from build123d import *
from OCP.BRepFilletAPI import BRepFilletAPI_MakeChamfer

# Parameters (mm, degrees)
SKETCH1_R                      = 20.575
SKETCH1_R_2                    = 18.575
BOSS_EXTRUDE1_DEPTH            = 20
BOSS_EXTRUDE2_START            = -1.95
SKETCH2_R                      = 35.575
SKETCH2_R_2                    = 20.575
BOSS_EXTRUDE2_DEPTH            = 1.95
CHAMFER2_SIZE                  = 2
CHAMFER2_SIZE2                 = 0.727940469
SKETCH3_W                      = 2
SKETCH3_H                      = 18
CUT_EXTRUDE1_DEPTH             = 0.8
CHAMFER3_SIZE                  = 2.197981936
CHAMFER3_SIZE_2                = 0.8
CIRPATTERN2_COUNT              = 6
CHAMFER3_OF_CIRPATTERN2_SIZE   = 2.197981936
CHAMFER3_OF_CIRPATTERN2_SIZE_2 = 0.8


with BuildPart() as part:
    # Sketch1 → Boss-Extrude1 (new body)
    with BuildSketch(Plane.XY):
        Circle(SKETCH1_R)
        Circle(SKETCH1_R_2, mode=Mode.SUBTRACT)
    extrude(amount=BOSS_EXTRUDE1_DEPTH)

    # Sketch2 → Boss-Extrude2 (add)
    with BuildSketch(Plane.XY.offset(20).offset(BOSS_EXTRUDE2_START)):
        Circle(SKETCH2_R)
        Circle(SKETCH2_R_2, mode=Mode.SUBTRACT)
    extrude(amount=BOSS_EXTRUDE2_DEPTH)

    # Chamfer2
    chamfer2_edges = [part.edges().sort_by_distance(p)[0] for p in [
        (-18.575, 0, 0),
        (-18.575, 0, 20),
    ]]
    chamfer2_side = [part.faces().sort_by_distance(p)[0] for p in [
        (-18.575, 0, 10),
    ]]
    chamfer(chamfer2_edges, length=CHAMFER2_SIZE, length2=CHAMFER2_SIZE2, reference=chamfer2_side[0])

    # Sketch3 → Cut-Extrude1 (cut)
    with BuildSketch(Plane.XY.offset(20)):
        with Locations((0, 27.575)):
            Rectangle(SKETCH3_W, SKETCH3_H)
    cut_extrude1 = extrude(amount=-CUT_EXTRUDE1_DEPTH, mode=Mode.SUBTRACT)

    # Chamfer3
    chamfer3_edges_1 = [part.edges().sort_by_distance(p)[0] for p in [
        (1, 27.418981343, 20),
    ]]
    chamfer3_side_1 = [part.faces().sort_by_distance(p)[0] for p in [
        (1.016, 27.418981343, 20),
    ]]
    chamfer3_edges_2 = [part.edges().sort_by_distance(p)[0] for p in [
        (-1, 27.418981343, 20),
    ]]
    chamfer3_side_2 = [part.faces().sort_by_distance(p)[0] for p in [
        (-1.016, 27.418981343, 20),
    ]]
    chamfer3 = BRepFilletAPI_MakeChamfer(part.part.solid().wrapped)
    for e in chamfer3_edges_1:
        chamfer3.Add(CHAMFER3_SIZE - 0.0001, CHAMFER3_SIZE_2 - 0.0001, e.wrapped, chamfer3_side_1[0].wrapped)
    for e in chamfer3_edges_2:
        chamfer3.Add(CHAMFER3_SIZE - 0.0001, CHAMFER3_SIZE_2 - 0.0001, e.wrapped, chamfer3_side_2[0].wrapped)
    add(Compound.cast(chamfer3.Shape()), mode=Mode.REPLACE)  # a hair under: the kernel refuses the full size

    # CirPattern2: Cut-Extrude1 ×6 about axis
    cirpattern2_axis = Axis((0, 0, 0), (0, 0, 1))
    for i in range(1, CIRPATTERN2_COUNT):
        add(cut_extrude1.rotate(cirpattern2_axis, i * 360 / CIRPATTERN2_COUNT), mode=Mode.SUBTRACT)

    # Chamfer3 of CirPattern2
    chamfer3_of_cirpattern2_edges_1 = [part.edges().sort_by_distance(p)[0] for p in [
        (-23.245534389, 14.575516075, 20),
    ]]
    chamfer3_of_cirpattern2_side_1 = [part.faces().sort_by_distance(p)[0] for p in [
        (-23.237534389, 14.589372482, 20),
    ]]
    chamfer3_of_cirpattern2_edges_2 = [part.edges().sort_by_distance(p)[0] for p in [
        (-24.245534389, 12.843465267, 20),
    ]]
    chamfer3_of_cirpattern2_side_2 = [part.faces().sort_by_distance(p)[0] for p in [
        (-24.245534389, 12.843465267, 19.984),
    ]]
    chamfer3_of_cirpattern2_edges_3 = [part.edges().sort_by_distance(p)[0] for p in [
        (-24.245534389, -12.843465267, 20),
    ]]
    chamfer3_of_cirpattern2_side_3 = [part.faces().sort_by_distance(p)[0] for p in [
        (-24.253534389, -12.829608861, 20),
    ]]
    chamfer3_of_cirpattern2_edges_4 = [part.edges().sort_by_distance(p)[0] for p in [
        (-23.245534389, -14.575516075, 20),
    ]]
    chamfer3_of_cirpattern2_side_4 = [part.faces().sort_by_distance(p)[0] for p in [
        (-23.245534389, -14.575516075, 19.984),
    ]]
    chamfer3_of_cirpattern2_edges_5 = [part.edges().sort_by_distance(p)[0] for p in [
        (-1, -27.418981343, 20),
    ]]
    chamfer3_of_cirpattern2_side_5 = [part.faces().sort_by_distance(p)[0] for p in [
        (-1.016, -27.418981343, 20),
    ]]
    chamfer3_of_cirpattern2_edges_6 = [part.edges().sort_by_distance(p)[0] for p in [
        (1, -27.418981343, 20),
    ]]
    chamfer3_of_cirpattern2_side_6 = [part.faces().sort_by_distance(p)[0] for p in [
        (1, -27.418981343, 19.984),
    ]]
    chamfer3_of_cirpattern2_edges_7 = [part.edges().sort_by_distance(p)[0] for p in [
        (23.245534389, -14.575516075, 20),
    ]]
    chamfer3_of_cirpattern2_side_7 = [part.faces().sort_by_distance(p)[0] for p in [
        (23.237534389, -14.589372482, 20),
    ]]
    chamfer3_of_cirpattern2_edges_8 = [part.edges().sort_by_distance(p)[0] for p in [
        (24.245534389, -12.843465267, 20),
    ]]
    chamfer3_of_cirpattern2_side_8 = [part.faces().sort_by_distance(p)[0] for p in [
        (24.245534389, -12.843465267, 19.984),
    ]]
    chamfer3_of_cirpattern2_edges_9 = [part.edges().sort_by_distance(p)[0] for p in [
        (24.245534389, 12.843465267, 20),
    ]]
    chamfer3_of_cirpattern2_side_9 = [part.faces().sort_by_distance(p)[0] for p in [
        (24.253534389, 12.829608861, 20),
    ]]
    chamfer3_of_cirpattern2_edges_10 = [part.edges().sort_by_distance(p)[0] for p in [
        (23.245534389, 14.575516075, 20),
    ]]
    chamfer3_of_cirpattern2_side_10 = [part.faces().sort_by_distance(p)[0] for p in [
        (23.245534389, 14.575516075, 19.984),
    ]]
    chamfer3_of_cirpattern2 = BRepFilletAPI_MakeChamfer(part.part.solid().wrapped)
    for e in chamfer3_of_cirpattern2_edges_1:
        chamfer3_of_cirpattern2.Add(CHAMFER3_OF_CIRPATTERN2_SIZE - 0.0001, CHAMFER3_OF_CIRPATTERN2_SIZE_2 - 0.0001, e.wrapped, chamfer3_of_cirpattern2_side_1[0].wrapped)
    for e in chamfer3_of_cirpattern2_edges_2:
        chamfer3_of_cirpattern2.Add(CHAMFER3_OF_CIRPATTERN2_SIZE_2 - 0.0001, CHAMFER3_OF_CIRPATTERN2_SIZE - 0.0001, e.wrapped, chamfer3_of_cirpattern2_side_2[0].wrapped)
    for e in chamfer3_of_cirpattern2_edges_3:
        chamfer3_of_cirpattern2.Add(CHAMFER3_OF_CIRPATTERN2_SIZE - 0.0001, CHAMFER3_OF_CIRPATTERN2_SIZE_2 - 0.0001, e.wrapped, chamfer3_of_cirpattern2_side_3[0].wrapped)
    for e in chamfer3_of_cirpattern2_edges_4:
        chamfer3_of_cirpattern2.Add(CHAMFER3_OF_CIRPATTERN2_SIZE_2 - 0.0001, CHAMFER3_OF_CIRPATTERN2_SIZE - 0.0001, e.wrapped, chamfer3_of_cirpattern2_side_4[0].wrapped)
    for e in chamfer3_of_cirpattern2_edges_5:
        chamfer3_of_cirpattern2.Add(CHAMFER3_OF_CIRPATTERN2_SIZE - 0.0001, CHAMFER3_OF_CIRPATTERN2_SIZE_2 - 0.0001, e.wrapped, chamfer3_of_cirpattern2_side_5[0].wrapped)
    for e in chamfer3_of_cirpattern2_edges_6:
        chamfer3_of_cirpattern2.Add(CHAMFER3_OF_CIRPATTERN2_SIZE_2 - 0.0001, CHAMFER3_OF_CIRPATTERN2_SIZE - 0.0001, e.wrapped, chamfer3_of_cirpattern2_side_6[0].wrapped)
    for e in chamfer3_of_cirpattern2_edges_7:
        chamfer3_of_cirpattern2.Add(CHAMFER3_OF_CIRPATTERN2_SIZE - 0.0001, CHAMFER3_OF_CIRPATTERN2_SIZE_2 - 0.0001, e.wrapped, chamfer3_of_cirpattern2_side_7[0].wrapped)
    for e in chamfer3_of_cirpattern2_edges_8:
        chamfer3_of_cirpattern2.Add(CHAMFER3_OF_CIRPATTERN2_SIZE_2 - 0.0001, CHAMFER3_OF_CIRPATTERN2_SIZE - 0.0001, e.wrapped, chamfer3_of_cirpattern2_side_8[0].wrapped)
    for e in chamfer3_of_cirpattern2_edges_9:
        chamfer3_of_cirpattern2.Add(CHAMFER3_OF_CIRPATTERN2_SIZE - 0.0001, CHAMFER3_OF_CIRPATTERN2_SIZE_2 - 0.0001, e.wrapped, chamfer3_of_cirpattern2_side_9[0].wrapped)
    for e in chamfer3_of_cirpattern2_edges_10:
        chamfer3_of_cirpattern2.Add(CHAMFER3_OF_CIRPATTERN2_SIZE_2 - 0.0001, CHAMFER3_OF_CIRPATTERN2_SIZE - 0.0001, e.wrapped, chamfer3_of_cirpattern2_side_10[0].wrapped)
    add(Compound.cast(chamfer3_of_cirpattern2.Shape()), mode=Mode.REPLACE)  # a hair under: the kernel refuses the full size


solid = part.part
Model file for the job. Use its own axes, mm. A direction names the side the tool comes from. Give positions to 0.01 mm unless a question says otherwise; leave off trailing zeros. Write each loop counter-clockwise with the first axis right and the second up, starting at its lowest first coordinate (ties: lowest second). Pieces come first, ordered by that corner, then holes. Notation, with made-up numbers: (-10.75, 2) -> (23.25, 2) arc R24 ccw to (23.25, 35) -> close; hole circle Ø11 at (64.25, -9). An arc over 180 degrees is marked (long way). Write item = value, one per line.
(1) Probe line 1 along Y through (x, z) = (0, 11) (3 decimals); line 2 along Z through (x, y) = (28.5, -15.5); line 3 along Z through (x, y) = (9, 29.5). List the from-to ranges inside material, lowest first.
Determined:
line_1 = -20.575 to -18.575, 18.575 to 20.575
line_2 = 18.05 to 19.2
line_3 = 18.05 to 20
(2) Mould opens along X. For faces 1 (the face through (-2.1, 27.2, 19.6)), 2 (the face through (11.06, 17.35, 8.9)), 3 (the face through (22.462, 15.41, 19.606)) say: released by +X, released by -X, zero draft, split by the parting line, or undercut.
Determined:
face_1 = undercut
face_2 = split by the parting line
face_3 = undercut
(3) Slice it at C-C, the plane z = 12.75. Give the cut face in (x, y) (3 decimals), then the cut area to 3 significant figures.
Determined:
outline = circle Ø41.15 at (0, 0); hole circle Ø37.15 at (0, 0)
area = 246 mm2
(4) Slice it at A-A, the plane y = 0. Give the cut face in (x, z) (3 decimals), then the cut area to 3 significant figures.
Determined:
outline = (-35.575, 18.05) -> (-20.575, 18.05) -> (-20.575, 0) -> (-19.303, 0) -> (-18.575, 2) -> (-18.575, 18) -> (-19.303, 20) -> (-35.575, 20) -> close; (18.575, 2) -> (19.303, 0) -> (20.575, 0) -> (20.575, 18.05) -> (35.575, 18.05) -> (35.575, 20) -> (19.303, 20) -> (18.575, 18) -> close
area = 136 mm2
(5) Slice it at B-B, the plane x = 0. Give the cut face in (y, z) (3 decimals), then the cut area to 3 significant figures.
Determined:
outline = (-35.575, 18.05) -> (-20.575, 18.05) -> (-20.575, 0) -> (-19.303, 0) -> (-18.575, 2) -> (-18.575, 18) -> (-19.012, 19.2) -> (-35.575, 19.2) -> close; (18.575, 2) -> (19.303, 0) -> (20.575, 0) -> (20.575, 18.05) -> (35.575, 18.05) -> (35.575, 19.2) -> (19.012, 19.2) -> (18.575, 18) -> close
area = 109 mm2
(6) Flat gauge pins, fed straight in: P1, Ø1.6, axis at x = 0, y = -28, coming from the +Z side; P2, Ø8, axis at x = -21, y = 11.5, coming from the +Z side; P3, Ø3, axis at y = -14.5, z = 17.5, coming from the -X side; P4, Ø3, axis at y = -24.5, z = 17, coming from the +X side. Where does each tip first touch, or does it go through?
Determined:
P1 = 19.2
P2 = 20
P3 = -33.07
P4 = 26.77
(7) Tool access for faces 4 (the face through (-22.477, 15.383, 19.594)), 5 (the face through (0, 27, 19.2)): list every direction of +Z, -Z, +X, -X, +Y, -Y with a clear straight run to the whole face (end or side of a thin tool).
Determined:
face_4 = +Z
face_5 = +Z, +Y, -Y
